from build123d import *


with BuildPart() as part:
    # Esquisse2 → Révolution1 (revolve)
    with BuildSketch(Plane(origin=(0, 0, 0), x_dir=(0, 0, -1), z_dir=(1, 0, 0)), mode=Mode.PRIVATE) as r_volution1_sk:
        Polygon((-6.5, 10.4), (-6.25, 10.4), (-6.25, 10.6), (6.25, 10.6), (6.25, 10.4), (6.5, 10.4), (6.5, 9.4), (6.25, 9.4), (6.25, 9.2), (-6.25, 9.2), (-6.25, 9.4), (-6.5, 9.4), align=None)
    revolve(r_volution1_sk.sketch.rotate(Axis((0, 0, 6.88356419), (0, 0, -1)), 90), axis=Axis((0, 0, 6.88356419), (0, 0, -1)))


solid = part.part
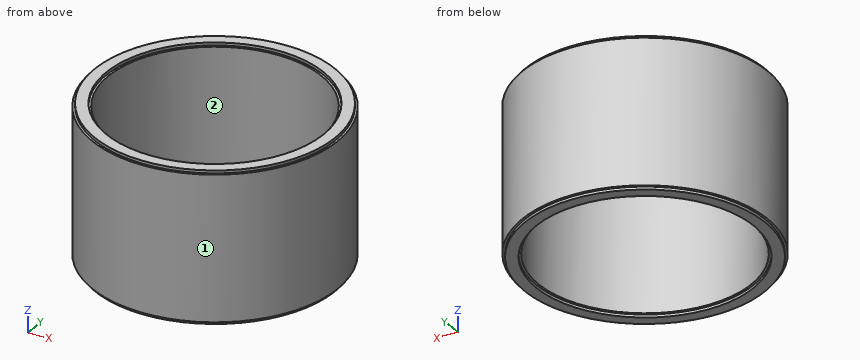
Geometry check sheet. Reference: the model listing, model coordinates, mm. Face numbers are marked on the shaded views. Give positions to 0.01 mm unless a question says otherwise; leave off trailing zeros. Order: outer loops, then holes, each group sorted by start corner. A loop starts at its lowest first (then second) coordinate and runs counter-clockwise, first axis right, second up. Notation, with made-up numbers: (-38, 40) - (20, 40) arc R10 ccw to (20, 57) - close; hole circle Ø10 at (14.25, 12.25). An arc over 180 degrees is marked (long way). Answer as a JSON object with one key per item and string values.
(1) Cross-section at A-A (x = 0). Record the cut outline in (y, z).
Report:
{"outline": "(-10.6, -6.25) - (-10.4, -6.25) - (-10.4, -6.5) - (-9.4, -6.5) - (-9.4, -6.25) - (-9.2, -6.25) - (-9.2, 6.25) - (-9.4, 6.25) - (-9.4, 6.5) - (-10.4, 6.5) - (-10.4, 6.25) - (-10.6, 6.25) - close; (9.2, -6.25) - (9.4, -6.25) - (9.4, -6.5) - (10.4, -6.5) - (10.4, -6.25) - (10.6, -6.25) - (10.6, 6.25) - (10.4, 6.25) - (10.4, 6.5) - (9.4, 6.5) - (9.4, 6.25) - (9.2, 6.25) - close"}
(2) Draft check along Y on the marked faces 1 and 2. Enter one of: released by +Y, released by -Y, zero draft, split by the parting line, or undercut.
Report:
{"face 1": "split by the parting line", "face 2": "undercut"}
(3) Cross-section at C-C (z = -2.25). Record the cut outline in (x, y).
Report:
{"outline": "circle Ø21.2 at (0, 0); hole circle Ø18.4 at (0, 0)"}
(4) Depth check by flat-ended pin: pin 1 Ø1 at (x, z) = (6.5, -4.5) entering from +Y; pin 2 Ø9.5 at (x, y) = (-4, -3) entering from -Z; pin 3 Ø2 at (x, z) = (7, 3) entering from -Y; pin 4 Ø6 at (x, z) = (-6, -3) entering from -Y. Enter the tip coordinate at first touch or a pass-through.
Report:
{"pin 1": "y = 8.74", "pin 2": "z = -6.5", "pin 3": "y = -8.74", "pin 4": "y = -10.17"}
(5) Material ranges on line 1 (X direction, y = 0.25, z = 5); line 2 (X direction, y = -8.25, z = -3.25); line 3 (Y direction, x = 3.25, z = -4), recorded low to high.
Report:
{"line 1": "-10.6 to -9.2, 9.2 to 10.6", "line 2": "-6.66 to -4.07, 4.07 to 6.66", "line 3": "-10.09 to -8.61, 8.61 to 10.09"}
